The model under review builds one solid part; all positions refer to its coordinate system, in mm. Face numbers are marked on the shaded views. A direction names the side the tool comes from. Round coordinates to 2 decimals unless told otherwise and drop trailing zeros. Order: outer loops, then holes, each group sorted by start corner. A loop starts at its lowest first (then second) coordinate and runs counter-clockwise, first axis right, second up.
1) Consider section B-B (y = 0.45). Give the boundary of the cut face in (x, z).
2) Clearance check with a flat-ended pin moving along its axis: P1, Ø1.5, axis at x = -4.5, y = 0.5, coming from the -Z side. State where the tip first meets the part, or that it passes through.
3) Mouldability with a two-part tool opening along X and no side actions: class the marked faces 3, 4 and 5 as pulls with the +X half, pulls with the -X half, needs draft (parallel to the pull), parting line crosses it, or undercut.
4) To check wall thickness, follow L1, parallel to X at y = 0.8, z = 0; L2, parallel to Y at x = -23.5, z = 2.75; L3, parallel to Z at x = -28.5, y = 1.05. State the ranges of each line that lie inside material, in increasing order.
5) Consider section C-C (x = -27.5). Give the boundary of the cut face in (y, z).
6) Machinability: for the marked faces 1 and 2, which of the approach directions +Z, -Z, +X, -X, +Y, -Y give a long, thin tool a straight path to every point of the face, cutting with its end or side? Answer none if there is none.
7) Consider section D-D (x = -11.5). Give the boundary of the cut face in (y, z).
8) Consider section A-A (z = 0). Give the boundary of the cut face in (x, y), then the cut area to 3 significant figures.
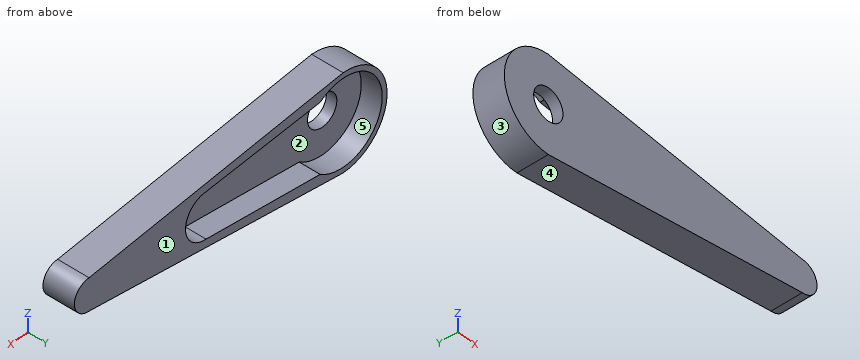
from build123d import *

# Parameters (mm, degrees)
SKETCH2_R           = 1.5
BOSS_EXTRUDE1_DEPTH = 1
BOSS_EXTRUDE2_DEPTH = 3


with BuildPart() as part:
    # Sketch2 → Boss-Extrude1 (new body)
    with BuildSketch(Plane(origin=(0, 0, 0), x_dir=(1, 0, 0), z_dir=(0, 1, 0))):
        with BuildLine():
            Line((-24.633695323, -3.234416395), (-12.961942578, -2.130426094))
            ThreePointArc((-12.961942578, -2.130426094), (-10.856533145, 0), (-12.961942578, 2.130426094))
            Line((-12.961942578, 2.130426094), (-24.633695323, 3.234416395))
            ThreePointArc((-24.633695323, 3.234416395), (-30.987107864, 0), (-24.633695323, -3.234416395))
        make_face()
        with Locations((-26.987107864, 0)):
            Circle(SKETCH2_R, mode=Mode.SUBTRACT)
    extrude(amount=BOSS_EXTRUDE1_DEPTH)

    # Sketch2<3> → Boss-Extrude2 (add)
    with BuildSketch(Plane(origin=(0, 0, 0), x_dir=(1, 0, 0), z_dir=(0, 1, 0))):
        with BuildLine():
            ThreePointArc((-26.987107864, 4.5), (-31.487107864, 0), (-26.987107864, -4.5))
            Line((-26.987107864, -4.5), (-0.987107864, -1.5))
            ThreePointArc((-0.987107864, -1.5), (0.512892136, 0), (-0.987107864, 1.5))
            Line((-0.987107864, 1.5), (-26.987107864, 4.5))
        make_face()
        with BuildLine():
            Line((-24.633695323, 3.234416395), (-12.961942578, 2.130426094))
            ThreePointArc((-12.961942578, 2.130426094), (-10.856533145, 0), (-12.961942578, -2.130426094))
            Line((-12.961942578, -2.130426094), (-24.633695323, -3.234416395))
            ThreePointArc((-24.633695323, -3.234416395), (-30.987107864, 0), (-24.633695323, 3.234416395))
        make_face(mode=Mode.SUBTRACT)
    extrude(amount=BOSS_EXTRUDE2_DEPTH)


solid = part.part
Answer below:
1. outline: (-26.99, -4.5) - (-0.99, -1.5) arc R1.5 ccw to (-0.99, 1.5) - (-26.99, 4.5) arc R4.5 ccw to start; hole circle Ø3 at (-26.99, 0)
2. P1: stops at z = -1.99
3. face 3: pulls with the -X half
3. face 4: pulls with the +X half
3. face 5: undercut
4. L1: x = -31.49 to -28.49, -25.49 to 0.51
4. L2: y = 0 to 1
4. L3: z = -4.24 to -3.7, 3.7 to 4.24
5. outline: (0, -4.47) - (3, -4.47) - (3, -3.97) - (1, -3.97) - (1, -1.41) - (0, -1.41) - close; (0, 1.41) - (1, 1.41) - (1, 3.97) - (3, 3.97) - (3, 4.47) - (0, 4.47) - close
6. face 1: +Z, -Z, +X, -X, +Y
6. face 2: +Y
7. outline: (0, -2.71) - (3, -2.71) - (3, -1.53) - (1, -1.53) - (1, 1.53) - (3, 1.53) - (3, 2.71) - (0, 2.71) - close
8. outline: (-31.49, 0) - (-28.49, 0) - (-28.49, 1) - (-30.99, 1) - (-30.99, 3) - (-31.49, 3) - close; (-25.49, 0) - (0.51, 0) - (0.51, 3) - (-10.86, 3) - (-10.86, 1) - (-25.49, 1) - close
8. area: 52.7 mm2
